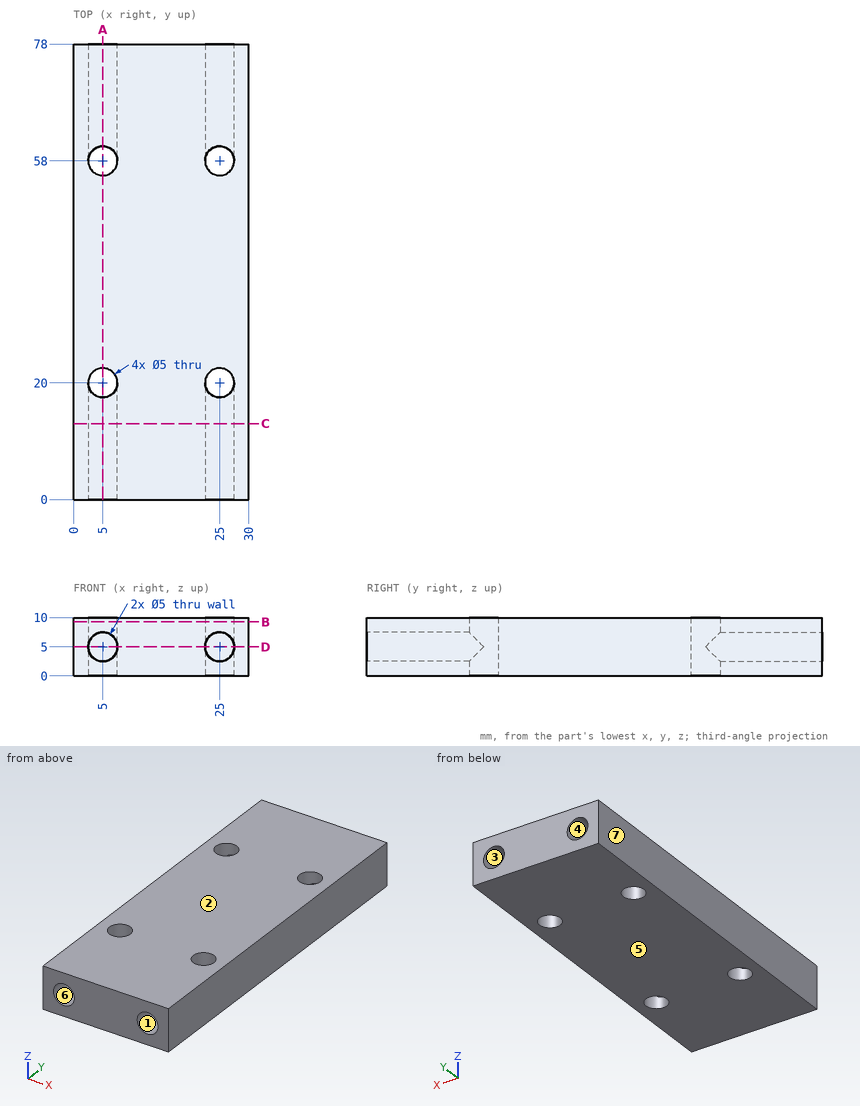
Answer from the drawing. Dimensions are ordinates in mm from the lowest x, y and z of the part. A direction names the side the tool comes from. Give positions to 0.01 mm unless a question says otherwise; leave off trailing zeros. Loops run counter-clockwise (first coordinate to the right, second up) from the corner with the lowest first, then second, coordinate; pieces in that order, holes last. Notation, with made-up numbers: (-39, 56.25) -> (3, 56.25) arc R28 ccw to (3, 95.25) -> close; hole circle Ø10 at (-17, 4). An arc over 180 degrees is marked (long way). Answer as CSV lines item,"result".
Item 1: Find section B-B on z = 9.25. Give the vertices of the cut face in (x, y), plus the area to 3 significant figures.
Returned:
outline,"(0, 0) -> (30, 0) -> (30, 78) -> (0, 78) -> close; hole circle Ø5 at (5, 20); hole circle Ø5 at (5, 58); hole circle Ø5 at (25, 20); hole circle Ø5 at (25, 58)"
area,"2,260 mm²"
Item 2: Find section C-C on y = 13. Give the vertices of the cut face in (x, z), plus the area to 3 significant figures.
Returned:
outline,"(0, 0) -> (30, 0) -> (30, 10) -> (0, 10) -> close; hole circle Ø5 at (5, 5); hole circle Ø5 at (25, 5)"
area,"261 mm²"
Item 3: Determine the mould class of the marked faces 4, 5, 6 and 7 for opening direction Z: +Z half, -Z half, draft (parallel to the pull), parting line (faces both ways), or undercut.
Returned:
face 4,"undercut"
face 5,"-Z half"
face 6,"undercut"
face 7,"draft"
Item 4: For the marked faces 1, 2 and 3, determine the directions among +Z, -Z, +X, -X, +Y, -Y from which every point of the face is accessible in a straight line to the end or side of a thin tool.
Returned:
face 1,"-Y"
face 2,"+Z, +X, -X, +Y, -Y"
face 3,"+Y"
Item 5: Find section A-A on x = 5. Give the vertices of the cut face in (y, z), plus the area to 3 significant figures.
Returned:
outline,"(0, 0) -> (17.5, 0) -> (17.5, 2.5) -> (0, 2.5) -> close; (0, 7.5) -> (17.5, 7.5) -> (17.5, 10) -> (0, 10) -> close; (22.5, 0) -> (55.5, 0) -> (55.5, 10) -> (22.5, 10) -> close; (60.5, 0) -> (78, 0) -> (78, 2.5) -> (60.5, 2.5) -> close; (60.5, 7.5) -> (78, 7.5) -> (78, 10) -> (60.5, 10) -> close"
area,"505 mm²"
Item 6: Consider line 1 (X direction, y = 12.5, z = 5); line 2 (Z direction, x = 5, y = 14.5); line 3 (X direction, y = 11.5, z = 7). Determine where each line is inside the solid, lowest interval first. Write a range as [from, to].
Returned:
line 1,"x = [0, 2.5], [7.5, 22.5], [27.5, 30]"
line 2,"z = [0, 2.5], [7.5, 10]"
line 3,"x = [0, 3.5], [6.5, 23.5], [26.5, 30]"
Item 7: Find section D-D on z = 5. Give the vertices of the cut face in (x, y).
Returned:
outline,"(0, 0) -> (2.5, 0) -> (2.5, 20) arc R2.5 cw to (7.5, 20) -> (7.5, 0) -> (22.5, 0) -> (22.5, 20) arc R2.5 cw to (27.5, 20) -> (27.5, 0) -> (30, 0) -> (30, 78) -> (27.5, 78) -> (27.5, 58) arc R2.5 cw to (22.5, 58) -> (22.5, 78) -> (7.5, 78) -> (7.5, 58) arc R2.5 cw to (2.5, 58) -> (2.5, 78) -> (0, 78) -> close"
Item 8: Each of these flat-tipped pins is pushed along its axis until it touches: pin 1 (1.5 mm diameter, centred on x = 3.5, z = 4.5, fed in from +Y); pin 2 (3 mm diameter, centred on x = 5, z = 5, fed in from -Y). Where does it stop, or does it pass through?
Returned:
pin 1,"stops at y = 56.91"
pin 2,"stops at y = 22"
